```python
from build123d import *

# Parameters (mm, degrees)
SKETCH1_W           = 304.8
SKETCH1_H           = 304.8
BOSS_EXTRUDE1_DEPTH = 6.35
CUT_EXTRUDE2_DEPTH  = 6.35
SKETCH3_R           = 1.9939
SKETCH3_R_2         = 1.3890625
CUT_EXTRUDE3_DEPTH  = 311.176538442


with BuildPart() as part:
    # Sketch1 → Boss-Extrude1 (new body)
    with BuildSketch(Plane(origin=(0, 0, 0), x_dir=(1, 0, 0), z_dir=(0, 1, 0))):
        with Locations((152.4, 152.4)):
            Rectangle(SKETCH1_W, SKETCH1_H)
    extrude(amount=BOSS_EXTRUDE1_DEPTH)

    # Sketch2 → Cut-Extrude2 (cut)
    with BuildSketch(Plane(origin=(0, 6.35, 0), x_dir=(1, 0, 0), z_dir=(0, 1, 0))):
        Polygon((57.15, 304.8), (57.15, 293.6875), (0, 293.6875), (0, 0), (304.8, 0), (304.8, 304.8), align=None)
    extrude(amount=-CUT_EXTRUDE2_DEPTH, mode=Mode.SUBTRACT)

    # Sketch3 → Cut-Extrude3 (cut, through all)
    with BuildSketch(Plane(origin=(0, 6.35, 0), x_dir=(1, 0, 0), z_dir=(0, 1, 0))):
        with Locations(Location((6.35, 299.24375, 0), (0, 0, 270))):
            Circle(SKETCH3_R)
        with Locations(Location((50.8, 299.24375, 0), (0, 0, 270))):
            Circle(SKETCH3_R_2)
        with Locations(Location((38.1, 299.24375, 0), (0, 0, 270))):
            Circle(SKETCH3_R_2)
    extrude(amount=-CUT_EXTRUDE3_DEPTH, mode=Mode.SUBTRACT)


solid = part.part
```
Part model, mm, in its own coordinate system. Give positions to 0.01 mm unless a question says otherwise; leave off trailing zeros. Write each loop counter-clockwise with the first axis right and the second up, starting at its lowest first coordinate (ties: lowest second). Pieces come first, ordered by that corner, then holes. Notation, with made-up numbers: (15, 18.5) -> (72, 18.5) arc R29 ccw to (72, 56.5) -> close; hole circle Ø1 at (79.25, 39). An arc over 180 degrees is marked (long way). Put each result on its own line as item: value. Start each with the question number.
Item 1: Cut at B-B (y = 1.75). List the corners of the cut face in (x, z).
Item 2: Cut at A-A (x = 6.35). List the corners of the cut face in (y, z).
Item 3: Pin check, flat tips, straight feed: pin 1 Ø1.7 at (x, z) = (38.1, -299.24) entering from -Y; pin 2 Ø3 at (y, z) = (1, -300) entering from -X. Stop position of each tip, or through.
Item 4: Wall check: L1, parallel to X at y = 4.75, z = -301; L2, parallel to X at y = 3.5, z = -298.5; L3, parallel to X at y = 5, z = -300.25. Give the ranges that are in metal, low to high. Write a range as [from, to].
Item 5: Pull direction X, two halves, no side cores. Call faces 1 (the face through (0, 3, -299)), 2 (the face through (57.15, 3, -299)), 3 (the face through (6.949, 3.219, -297.342)), 4 (the face through (28, 3, -304.8)): pulls with the +X half, pulls with the -X half, needs draft (parallel to the pull), parting line crosses it, or undercut.
Item 6: Cut at D-D (x = 38.1). List the corners of the cut face in (y, z), then the cut area to 3 significant figures.
Item 7: Cut at C-C (z = -298.5). List the corners of the cut face in (x, y).
Answer list:
1. outline: (0, -304.8) -> (57.15, -304.8) -> (57.15, -293.69) -> (0, -293.69) -> close; hole circle Ø3.99 at (6.35, -299.24); hole circle Ø2.78 at (38.1, -299.24); hole circle Ø2.78 at (50.8, -299.24)
2. outline: (0, -304.8) -> (6.35, -304.8) -> (6.35, -301.24) -> (0, -301.24) -> close; (0, -297.25) -> (6.35, -297.25) -> (6.35, -293.69) -> (0, -293.69) -> close
3. pin 1: passes through
3. pin 2: stops at x = 0
4. L1: x = [0, 5.41], [7.29, 57.15]
4. L2: x = [0, 4.5], [8.2, 36.93], [39.27, 49.63], [51.97, 57.15]
4. L3: x = [0, 4.63], [8.07, 37.14], [39.06, 49.84], [51.76, 57.15]
5. face 1: pulls with the -X half
5. face 2: pulls with the +X half
5. face 3: undercut
5. face 4: needs draft
6. outline: (0, -304.8) -> (6.35, -304.8) -> (6.35, -300.63) -> (0, -300.63) -> close; (0, -297.85) -> (6.35, -297.85) -> (6.35, -293.69) -> (0, -293.69) -> close
6. area: 52.9 mm2
7. outline: (0, 0) -> (4.5, 0) -> (4.5, 6.35) -> (0, 6.35) -> close; (8.2, 0) -> (36.93, 0) -> (36.93, 6.35) -> (8.2, 6.35) -> close; (39.27, 0) -> (49.63, 0) -> (49.63, 6.35) -> (39.27, 6.35) -> close; (51.97, 0) -> (57.15, 0) -> (57.15, 6.35) -> (51.97, 6.35) -> close
